```python
from build123d import *

# Parameters (mm, degrees)
SKETCH_W     = 31.75
SKETCH_H     = 31.75
SKETCH_W_2   = 26.2128
SKETCH_H_2   = 26.2128
PAD_DEPTH    = 457.2
POCKET_DEPTH = 31.75


with BuildPart() as part:
    # Sketch → Pad (new body)
    with BuildSketch(Plane.XZ):
        Rectangle(SKETCH_W, SKETCH_H)
        Rectangle(SKETCH_W_2, SKETCH_H_2, mode=Mode.SUBTRACT)
    extrude(amount=PAD_DEPTH)

    # Sketch001 → Pocket (cut)
    with BuildSketch(Plane(origin=(0, 0, 15.875), x_dir=(-1, 0, 0), z_dir=(0, 0, 1))):
        Polygon((15.875, 457.2), (-15.875, 457.2), (-15.875, 425.45), align=None)
    extrude(amount=-POCKET_DEPTH, mode=Mode.SUBTRACT)


solid = part.part
```
Could you check a few things on this model? Use its own coordinates, in mm. A direction names the side the tool comes from. Round coordinates to 2 decimals unless told otherwise and drop trailing zeros. Loops run counter-clockwise (first coordinate to the right, second up) from the corner with the lowest first, then second, coordinate; pieces in that order, holes last.
Q1. For P1, Ø3, axis at x = 10.5, z = -1.5, coming from the -Y side; P2, Ø5, axis at x = 4.5, z = 12.5, coming from the -Y side, each with a flat end and sliding along its axis, tell me the tip position at first contact or that it passes through.
Q2. Please list where these lines run through material, in increasing order: L1, parallel to X at y = -334, z = 12 (3 decimals); L2, parallel to Y at x = 15, z = 13.5 (3 decimals).
Q3. I want a section at C-C (x = 0). Write out the boundary of the cut face in (y, z) (3 decimals), and give its area (3 significant figures).
Q4. I want a section at B-B (y = -364). Write out the boundary of the cut face in (x, z) (3 decimals), and give its area (3 significant figures).
Q5. Thinking about a two-plate mould opening in Z: for faces 3 (the flat face through (13.106, -211, 0)), 4 (the flat face through (0, -225, -15.875)), 5 (the flat face through (15.875, -210, 0)), which applies, pulls with the +Z half, pulls with the -Z half, needs draft (parallel to the pull), parting line crosses it, or undercut?
Q6. I want a section at A-A (z = -2.5). Write out the boundary of the cut face in (x, y) (3 decimals), and give its area (3 significant figures).
Q7. On a 3-axis mill with a long thin cutter (end or side, diameter ignored), from which of +Z, -Z, +X, -X, +Y, -Y can I reach the whole of each face in a straight line? I mean faces 1 (the flat face through (0.222, -441.103, -13.889)), 2 (the flat face through (0, -224, -13.106)). Say none if no direction works.
Answer below:
1. P1: passes through
1. P2: stops at y = -439.25
2. L1: x = -15.875 to -13.106, 13.106 to 15.875
2. L2: y = -426.325 to 0
3. outline: (-441.325, -15.875) - (0, -15.875) - (0, -13.106) - (-441.325, -13.106) - close; (-441.325, 13.106) - (0, 13.106) - (0, 15.875) - (-441.325, 15.875) - close
3. area: 2,440 mm2
4. outline: (-15.875, -15.875) - (15.875, -15.875) - (15.875, 15.875) - (-15.875, 15.875) - close; hole (-13.106, -13.106) - (13.106, -13.106) - (13.106, 13.106) - (-13.106, 13.106) - close
4. area: 321 mm2
5. face 3: undercut
5. face 4: pulls with the -Z half
5. face 5: needs draft
6. outline: (-15.875, -457.2) - (-13.106, -454.431) - (-13.106, 0) - (-15.875, 0) - close; (13.106, -428.219) - (15.875, -425.45) - (15.875, 0) - (13.106, 0) - close
6. area: 2,440 mm2
7. face 1: +Z, -Z, +X, -Y
7. face 2: +Y, -Y
